Input: part model. Units: mm. Frame: model coordinates. A direction names the side the tool comes from. Give positions to 0.01 mm unless a question says otherwise; leave off trailing zeros. Loops run counter-clockwise (first coordinate to the right, second up) from the corner with the lowest first, then second, coordinate; pieces in that order, holes last. Notation, with made-up numbers: (24, 62.5) - (56, 62.5) arc R21 cw to (56, 91.5) - close; hole circle Ø3 at (35, -9.75). An arc over 180 degrees is marked (long way). Answer as a JSON object with one key per item and string values. Group by question number.
(1) Pin query (flat end, axial travel): P1, Ø3, axis at y = 2, z = -27, coming from the +X side; P2, Ø9, axis at x = 0, z = -63.375, coming from the -Y side; P3, Ø4, axis at x = -15.5, z = 26.875, coming from the -Y side; P4, Ø1.5, axis at y = 1.5, z = -54, coming from the -X side. Return the tip coordinate at first contact, or that it passes through.
(2) Section query C-C (z = -42). Return loops of the section in (x, y), plus the area to 3 significant figures.
(3) Access query for faces 1 (the cylindrical face through (2.69, 3.13, -67.59)), 2 (the flat face through (10, 3, -34)). Directions: +Z, -Z, +X, -X, +Y, -Y. A direction counts if a zero-diameter tool reaches every point of the face in a straight line with its end or side. Return the directions, or none.
(4) Material intervals for L1, parallel to Z at x = 0, y = 3 (3 decimals); L2, parallel to Z at x = -16, y = 2.5 (3 decimals); L3, parallel to X at y = 4.75, z = 57, sorted ascending.
(5) Mould query, pull axis X, two halves, no side actions, for faces 3 (the flat face through (0, 0, 8)), 4 (the cylindrical face through (14.394, 3.131, 56.861)), 5 (the flat face through (-10, 3, -33)). Classes: +X half, -X half, draft (parallel to the pull), parting line (faces both ways), or undercut.
(6) Section query A-A (x = 0). Return loops of the section in (y, z) (3 decimals).
(7) Section query B-B (y = 3.75). Return loops of the section in (x, z) (3 decimals).
(8) Section query D-D (x = -15.5). Return loops of the section in (y, z) (3 decimals), plus the area to 3 significant figures.
```python
from build123d import *

# Parameters (mm, degrees)
SKETCH1_R           = 5
SKETCH1_R_2         = 1.5
SKETCH1_R_3         = 2.5
BOSS_EXTRUDE1_DEPTH = 6.35


with BuildPart() as part:
    # Sketch1 → Boss-Extrude1 (new body)
    with BuildSketch(Plane(origin=(0, 0, 0), x_dir=(1, 0, 0), z_dir=(0, 1, 0))):
        Polygon((-10, -9.622405772), (-10, 76.625), (10, 76.625), (10, -9.622405772), (22.5, -18.375), (22.5, -63.375), (0, -63.375), (-22.5, -63.375), (-22.5, -18.375), align=None)
        with Locations((0, 63.375)):
            Circle(SKETCH1_R, mode=Mode.SUBTRACT)
        with Locations((-15.5, -26.875)):
            Circle(SKETCH1_R_2, mode=Mode.SUBTRACT)
        with Locations((15.5, -26.875)):
            Circle(SKETCH1_R_2, mode=Mode.SUBTRACT)
        with Locations((15.5, -57.875)):
            Circle(SKETCH1_R_2, mode=Mode.SUBTRACT)
        with Locations((-15.5, -57.875)):
            Circle(SKETCH1_R_2, mode=Mode.SUBTRACT)
        with Locations((0, -42.375)):
            Circle(SKETCH1_R_3, mode=Mode.SUBTRACT)
    extrude(amount=BOSS_EXTRUDE1_DEPTH)


solid = part.part
```
Recorded:
{
 "1": {"P1": "stops at x = 10", "P2": "passes through", "P3": "stops at y = 0", "P4": "stops at x = -10"},
 "2": {"outline": "(-10, 0) - (10, 0) - (10, 6.35) - (-10, 6.35) - close", "area": "127 mm^2"},
 "3": {"face 1": "+Y, -Y", "face 2": "-Z, +X, +Y, -Y"},
 "4": {"L1": "z = -76.625 to -68.375, -58.375 to 39.875, 44.875 to 63.375", "L2": "z = 13.824 to 25.461, 28.289 to 56.461, 59.289 to 63.375", "L3": "x = -22.5 to -16.72, -14.28 to 14.28, 16.72 to 22.5"},
 "5": {"face 3": "draft", "face 4": "undercut", "face 5": "-X half"},
 "6": {"outline": "(0, -76.625) - (6.35, -76.625) - (6.35, -68.375) - (0, -68.375) - close; (0, -58.375) - (6.35, -58.375) - (6.35, 39.875) - (0, 39.875) - close; (0, 44.875) - (6.35, 44.875) - (6.35, 63.375) - (0, 63.375) - close"},
 "7": {"outline": "(-22.5, 18.375) - (-10, 9.622) - (-10, -76.625) - (10, -76.625) - (10, 9.622) - (22.5, 18.375) - (22.5, 63.375) - (-22.5, 63.375) - close; hole circle Ø3 at (-15.5, 26.875); hole circle Ø3 at (-15.5, 57.875); hole circle Ø10 at (0, -63.375); hole circle Ø5 at (0, 42.375); hole circle Ø3 at (15.5, 26.875); hole circle Ø3 at (15.5, 57.875)"},
 "8": {"outline": "(0, 13.474) - (6.35, 13.474) - (6.35, 25.375) - (0, 25.375) - close; (0, 28.375) - (6.35, 28.375) - (6.35, 56.375) - (0, 56.375) - close; (0, 59.375) - (6.35, 59.375) - (6.35, 63.375) - (0, 63.375) - close", "area": "279 mm^2"}
}
